```python
from build123d import *

# Parameters (mm, degrees)
F0_R     = 12.5
F0_R_2   = 6
F2_DEPTH = 25
F3_DEPTH = 12.5
F4_R     = 7.5
F6_R     = 6
F7_DEPTH = 25


with BuildPart() as f2:
    # F0 (on Top) → F2 (new body)
    with BuildSketch(Plane.XY):
        Circle(F0_R)
        Circle(F0_R_2, mode=Mode.SUBTRACT)
    extrude(amount=F2_DEPTH)



with BuildPart() as f3:
    # F0 (on Top) → F3 (new body, symmetric)
    with BuildSketch(Plane.XY):
        with Locations((150, 0)):
            Circle(F0_R)
        with Locations((150, 0)):
            Circle(F0_R_2, mode=Mode.SUBTRACT)
    extrude(amount=F3_DEPTH, both=True)


with BuildPart() as f2_1:
    add(f2.part)

    add(f3.part)  # F5 merges F3
    # F5: sweep along a path in F1
    with BuildLine(Plane.XZ) as f5_path:
        Line((0, 12), (21.4128675194, 12))
        ThreePointArc((21.4128675194, 12), (24.9936063711, 11.8930572711), (28.5615807565, 11.5726103092))
        Line((28.5615807565, 11.5726103092), (121.4384192435, 0.4273896908))
        ThreePointArc((121.4384192435, 0.4273896908), (125.0063936289, 0.1069427289), (128.5871324806, 0))
        Line((128.5871324806, 0), (150, 0))
    # F4 (on Right) → F5 (sweep)
    with BuildSketch(Plane.YZ):
        with Locations((0, 12)):
            Circle(F4_R)
    sweep(path=f5_path.line)

    # F6 (on Top) → F7 (cut, symmetric)
    with BuildSketch(Plane.XY):
        Circle(F6_R)
        with Locations((150, 0)):
            Circle(F6_R)
    extrude(amount=F7_DEPTH, both=True, mode=Mode.SUBTRACT)


solid = f2_1.part
```
Geometry: final body of the model. Coordinates: model frame, mm. A direction names the side the tool comes from. Give positions to 0.01 mm unless a question says otherwise; leave off trailing zeros. Write each loop counter-clockwise with the first axis right and the second up, starting at its lowest first coordinate (ties: lowest second). Pieces come first, ordered by that corner, then holes.
1. Section query A-A, the plane x = 150. Return loops of the section in (y, z), then the cut area to 3 significant figures.
2. Line query: probe 1 along Y at (x, z) = (0, 6); probe 2 along X at (y, z) = (2.75, 6); probe 3 along Z at (x, y) = (141, -5). Output: solid intervals per line, ascending.
3. Pin query (flat end, axial travel): P1, Ø8, axis at x = 56.5, z = -2, coming from the +Y side; P2, Ø5, axis at x = 9, z = 2, coming from the +Y side; P3, Ø10, axis at x = 101.5, y = 5.5, coming from the -Z side. Return the tip coordinate at first contact, or that it passes through.
4. Reachability of faces 4 (the flat face through (155.4, 3, 12.5)), 5 (the cylindrical face through (15.786, 4.032, 18.324)), 6 (the flat face through (-3, -5.4, 25)) from +Z, -Z, +X, -X, +Y, -Y: full face, straight path, thin tool, end or side. Return the list, or none.
5. Section query C-C, the plane y = 9.75. Return loops of the section in (x, z), then the cut area to 3 significant figures.
6. Section query D-D, the plane z = 21. Return loops of the section in (x, y), then the cut area to 3 significant figures.
7. Section query B-B, the plane y = 0. Return loops of the section in (x, z).
8. Draft query along Y for faces 1 (the cylindrical face through (145.24, -3.65, -0.18)), 2 (the cylindrical face through (161.923, 3.755, 0.175)), 3 (the flat face through (-3, -5.4, 0)). Return one class per face: released by +Y, released by -Y, zero draft, split by the parting line, or undercut.
Computed:
1. outline: (-12.5, -12.5) - (-6, -12.5) - (-6, 12.5) - (-12.5, 12.5) - close; (6, -12.5) - (12.5, -12.5) - (12.5, 12.5) - (6, 12.5) - close
1. area: 325 mm2
2. probe 1: y = -12.5 to -6, 6 to 12.5
2. probe 2: x = -12.19 to -5.33, 5.33 to 144.67, 155.33 to 162.19
2. probe 3: z = -12.5 to 12.5
3. P1: stops at y = 4.3
3. P2: stops at y = 10.68
3. P3: stops at z = -4.95
4. face 4: +Z, +X, +Y, -Y
4. face 5: none
4. face 6: +Z, +X, -X, +Y, -Y
5. outline: (-7.82, 0) - (7.82, 0) - (7.82, 25) - (-7.82, 25) - close; (142.18, -12.5) - (157.82, -12.5) - (157.82, 12.5) - (142.18, 12.5) - close
5. area: 782 mm2
6. outline: circle Ø25 at (0, 0); hole circle Ø12 at (0, 0)
6. area: 378 mm2
7. outline: (-12.5, 0) - (-6, 0) - (-6, 25) - (-12.5, 25) - close; (6, 0) - (12.5, 0) - (12.5, 4.5) - (21.41, 4.5) arc R52.5 cw to (27.67, 4.13) - (120.54, -7.02) arc R67.5 ccw to (128.59, -7.5) - (137.5, -7.5) - (137.5, -12.5) - (144, -12.5) - (144, 12.5) - (137.5, 12.5) - (137.5, 7.5) - (128.59, 7.5) arc R52.5 cw to (122.33, 7.87) - (29.46, 19.02) arc R67.5 ccw to (21.41, 19.5) - (12.5, 19.5) - (12.5, 25) - (6, 25) - close; (156, -12.5) - (162.5, -12.5) - (162.5, 12.5) - (156, 12.5) - close
8. face 1: undercut
8. face 2: split by the parting line
8. face 3: zero draft
